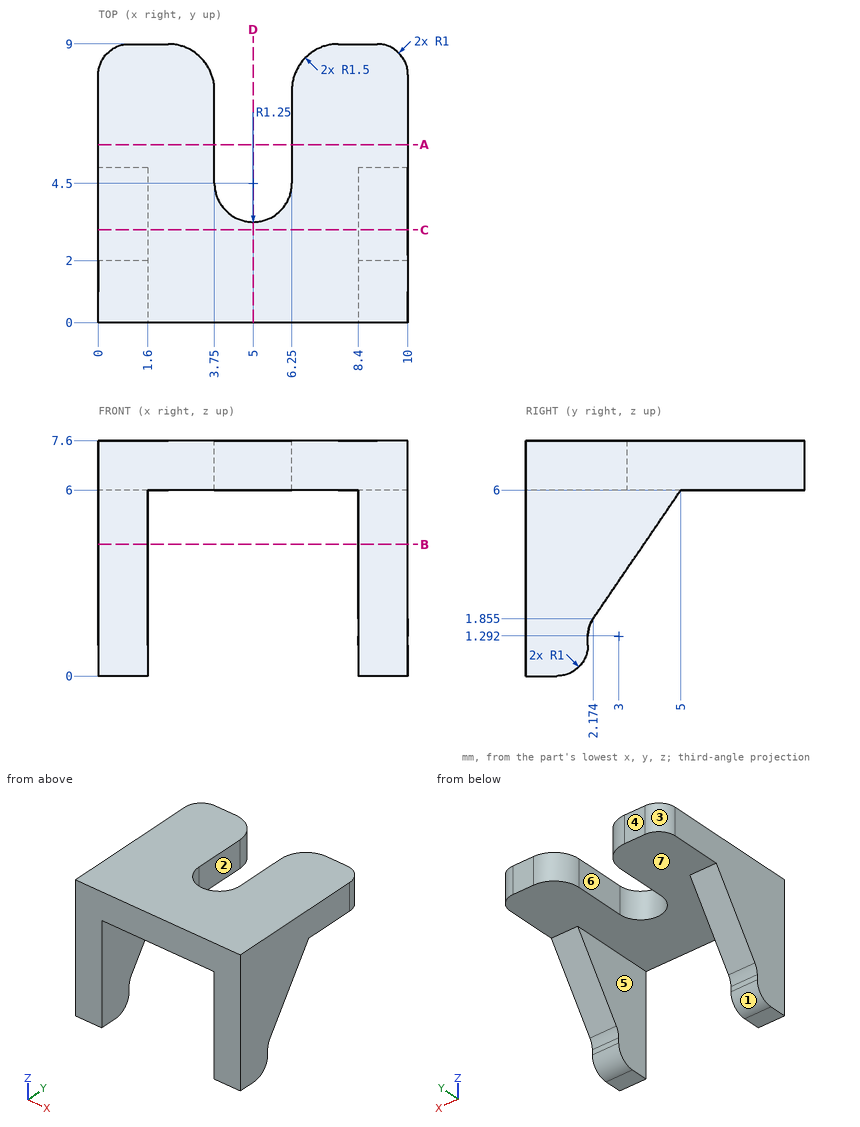
The figure shows three views and two pictorial views of one solid part (mm, origin at its lowest corner). Answer the questions. A direction names the side the tool comes from. Round coordinates to 2 decimals unless told otherwise and drop trailing zeros. Order: outer loops, then holes, each group sorted by start corner. A loop starts at its lowest first (then second) coordinate and runs counter-clockwise, first axis right, second up. Notation, with made-up numbers: (49.5, 19) -> (76.5, 19) arc R29 ccw to (76.5, 49) -> close; hole circle Ø5 at (-2.75, -7.75). An arc over 180 degrees is marked (long way). Put each result on its own line as item: value.
Q1. Section B-B, the plane z = 4.25 is taken. Write down the section's boundary in (x, y).
Results list:
outline: (0, 0) -> (1.6, 0) -> (1.6, 3.81) -> (0, 3.81) -> close; (8.4, 0) -> (10, 0) -> (10, 3.81) -> (8.4, 3.81) -> close
Q2. Which of the six approach directions +Z, -Z, +X, -X, +Y, -Y give full straight-line access (tool end or side, diameter ignored) to the marked faces 4, 5, 6 and 7?
Results list:
face 4: +Z, -Z, +X, -X, +Y
face 5: -Z, +Y, -Y
face 6: +Z, -Z, +Y
face 7: -Z, +Y
Q3. Section C-C, the plane y = 3 is taken. Write down the section's boundary in (x, z).
Results list:
outline: (0, 3.07) -> (1.6, 3.07) -> (1.6, 6) -> (8.4, 6) -> (8.4, 3.07) -> (10, 3.07) -> (10, 7.6) -> (0, 7.6) -> close
Q4. Section A-A, the plane y = 5.75 is taken. Write down the section's boundary in (x, z), and give its area (3 significant figures).
Results list:
outline: (0, 6) -> (3.75, 6) -> (3.75, 7.6) -> (0, 7.6) -> close; (6.25, 6) -> (10, 6) -> (10, 7.6) -> (6.25, 7.6) -> close
area: 12.0 mm^2
Q5. Section D-D, the plane x = 5 is taken. Write down the section's boundary in (y, z).
Results list:
outline: (0, 6) -> (3.25, 6) -> (3.25, 7.6) -> (0, 7.6) -> close
Q6. Consider line 1 along X through (y, z) = (2.75, 2.75); line 2 along X through (y, z) = (7, 6.5); line 3 along Z through (x, y) = (2.5, 4). Determine where each line is inside the solid, lowest interval first.
Results list:
line 1: 0 to 1.6, 8.4 to 10
line 2: 0 to 3.75, 6.25 to 10
line 3: 6 to 7.6
Q7. Determine the mould class of the marked faces 1, 2 and 3 for opening direction X: pulls with the +X half, pulls with the -X half, needs draft (parallel to the pull), parting line crosses it, or undercut.
Results list:
face 1: needs draft
face 2: undercut
face 3: pulls with the -X half
